from build123d import *

# Parameters (mm, degrees)
F1_DEPTH = 17.78
F3_DEPTH = 50.8
F5_DEPTH = 76.2
F7_DEPTH = 177.8
F8_DEPTH = 177.8


# Not quite as in the source:
# - a feature names something its author has since deleted; it is built from what else it names


with BuildPart() as f1:
    # F0 (on Top) → F1 (new body)
    with BuildSketch(Plane.XY):
        Polygon((-9.4930937983, 27.7505766331), (-28.7792512331, 5.6540279267), (-19.2861574348, -22.0965487064), (9.4930937983, -27.7505766331), (28.7792512331, -5.6540279267), (19.2861574348, 22.0965487064), align=None)
    extrude(amount=F1_DEPTH)

    # F2 (on face) → F3 (join)
    with BuildSketch(Plane.XY.offset(17.78)):
        Polygon((-1.5908913392, 23.4257021287), (-23.4257021287, -1.5908913392), (1.5908913392, -23.4257021287), (23.4257021287, 1.5908913392), align=None)
    extrude(amount=F3_DEPTH)

    # F4 (on face) → F5 (cut)
    with BuildSketch(Plane(origin=(-10.9174053947, -12.508296734, 0), x_dir=(0.7533926187, -0.6575709559, 0), z_dir=(-0.6575709559, -0.7533926187, 0))):
        with BuildLine():
            Line((0, 48.7790480256), (13.0695169792, 32.4794128537))
            Line((13.0695169792, 32.4794128537), (8.2184774801, 17.78))
            Line((8.2184774801, 17.78), (16.6026271336, 17.78))
            Line((16.6026271336, 17.78), (16.6026271336, 68.58))
            Line((16.6026271336, 68.58), (-16.6026271336, 68.58))
            Line((-16.6026271336, 68.58), (-16.6026271336, 17.78))
            Line((-16.6026271336, 17.78), (-9.5075005665, 17.78))
            ThreePointArc((-9.5075005665, 17.78), (-11.8387691089, 20.1965691968), (-13.1141533635, 23.3026945488))
            ThreePointArc((-13.1141533635, 23.3026945488), (-15.1729749394, 35.6082188112), (-14.361799588, 48.0583862079))
            ThreePointArc((-14.361799588, 48.0583862079), (-4.2065001242, 63.2907896054), (14.0689240854, 64.3701831512))
            Line((14.0689240854, 64.3701831512), (13.6791784316, 44.722918421))
            Line((13.6791784316, 44.722918421), (7.8148273751, 44.722918421))
            Line((7.8148273751, 44.722918421), (1.6052529907, 50.0661861116))
            Line((1.6052529907, 50.0661861116), (0, 48.7790480256))
        make_face()
    extrude(amount=-F5_DEPTH, mode=Mode.SUBTRACT)

    # F6 (on face) → F7 (cut)
    with BuildSketch(Plane(origin=(-10.9174053947, -12.508296734, 0), x_dir=(0.7533926187, -0.6575709559, 0), z_dir=(-0.6575709559, -0.7533926187, 0))):
        Polygon((8.6703589186, 57.2541877627), (6.4581842162, 59.0407550335), (6.4581842162, 56.6472448409), (8.6703589186, 54.8606775701), align=None)
    extrude(amount=-F7_DEPTH, mode=Mode.SUBTRACT)

    # F6 (on face) → F8 (cut)
    with BuildSketch(Plane(origin=(-10.9174053947, -12.508296734, 0), x_dir=(0.7533926187, -0.6575709559, 0), z_dir=(-0.6575709559, -0.7533926187, 0))):
        Polygon((8.6703589186, 57.2541877627), (6.4581842162, 59.0407550335), (6.4581842162, 56.6472448409), (8.6703589186, 54.8606775701), align=None)
    extrude(amount=-F8_DEPTH, mode=Mode.SUBTRACT)


solid = f1.part
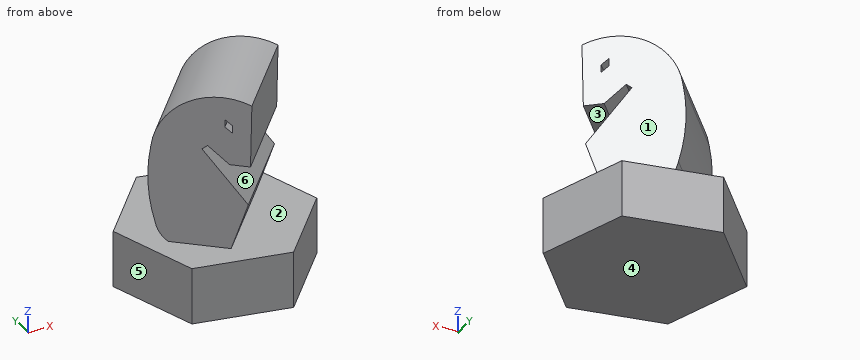
Work out the finished part from the listing and answer in its coordinate system (mm). Face numbers are marked on the shaded views. A direction names the side the tool comes from. Give positions to 0.01 mm unless a question says otherwise; leave off trailing zeros. Order: outer loops, then holes, each group sorted by start corner. A loop starts at its lowest first (then second) coordinate and runs counter-clockwise, first axis right, second up. Notation, with made-up numbers: M 13.5,56 L 41.5,56 A13 ccw 41.5,72 Z; hole C 13,3.25 d11. An arc over 180 degrees is marked long. Return JSON: item names as keys, results as strings.
Q1. The mould has two halves that part along Z. Classify the marked faces 4, 5 and 6: pulls with the +Z half, pulls with the -Z half, needs draft (parallel to the pull), parting line crosses it, or undercut.
Answer below:
{"face 4": "pulls with the -Z half", "face 5": "needs draft", "face 6": "undercut"}
Q2. Which of the six approach directions +Z, -Z, +X, -X, +Y, -Y give full straight-line access (tool end or side, diameter ignored) to the marked faces 1, 2 and 3?
Answer below:
{"face 1": "+Z, +X, +Y", "face 2": "none", "face 3": "+X, -Y"}
Q3. Each of these flat-tipped pins is pushed along its axis until it touches: pin 1 (21 mm diameter, centred on x = 7.5, y = -11.5, fed in from -Z); pin 2 (2 mm diameter, centred on x = 9, z = 36, fed in from +Y); pin 3 (8 mm diameter, centred on x = 11.5, z = 40.5, fed in from -Y); pin 4 (4 mm diameter, centred on y = 22, z = 8, fed in from -X). Where does it stop, or does it pass through?
Answer below:
{"pin 1": "stops at z = 0", "pin 2": "stops at y = 15.05", "pin 3": "stops at y = -3.61", "pin 4": "stops at x = -16.26"}
Q4. Find section B-B, the plane z = 28.5. Write down the section's boundary in (x, y).
Answer below:
{"outline": "M -21.72,-3.08 L -2.06,-20.24 L 19.77,4.78 L 0.11,21.94 Z"}
Q5. Find the intervals of material crossed by line 1 along Z through (x, y) = (7.5, -3.5); line 2 along Z through (x, y) = (5, -1); line 3 along Z through (x, y) = (-8.5, -13.5), in increasing order. Write a range as [from, to].
Answer below:
{"line 1": "z = [0, 38.86], [44.72, 55.44], [57.83, 65.92]", "line 2": "z = [0, 43.26], [47.64, 65.95]", "line 3": "z = [0, 45.69], [49.32, 65.71]"}
Q6. Find section A-A, the plane x = 13.5. State how many separate pieces and enclosed holes the cut face has, and give its area (3 significant figures).
Answer below:
{"separate pieces": "2", "enclosed holes": "1", "area": "1,390 mm^2"}
Q7. Find section C-C, the plane x = 22.5. Write down the section's boundary in (y, z).
Answer below:
{"outline": "M -12.85,0 L 12.7,0 L 12.7,17.78 L -12.85,17.78 Z"}
